Study the drawing (mm; zero at the part's minimum x, y, z) and answer. A direction names the side the tool comes from. Give positions to 0.01 mm unless a question says otherwise; leave off trailing zeros. Order: outer loops, then holes, each group sorted by start corner. A loop starts at its lowest first (then second) coordinate and runs counter-clockwise, first axis right, second up.
Item 1: Which of the six approach directions +Z, -Z, +X, -X, +Y, -Y give full straight-line access (tool end or side, diameter ignored) to the marked faces 1, 2 and 3?
Item 2: Find the intervals of material crossed by line 1 along Y through (x, z) = (3.5, 12.7); line 2 along Z through (x, y) = (3.25, 25.4); line 3 along Z through (x, y) = (17, 3), in increasing order.
Item 3: A cutting plane is placed at A-A (y = 25.4). Write down the section's boundary in (x, z), plus the area to 3 significant figures.
Item 4: A cutting plane is placed at B-B (x = 3.75). State how many separate pieces and enclosed holes the cut face has, plus the area to 3 significant figures.
Item 5: Given pin 1 Ø4 at (y, z) = (38.1, 12.7) entering from -X; pin 2 Ø6.5 at (x, z) = (12.5, 11.5) entering from -Y; pin 3 Ø7.5 at (x, z) = (16, 15) entering from +Y, each flat-ended and moving along its own axis, determine where each tip first touches the part or whether it passes through.
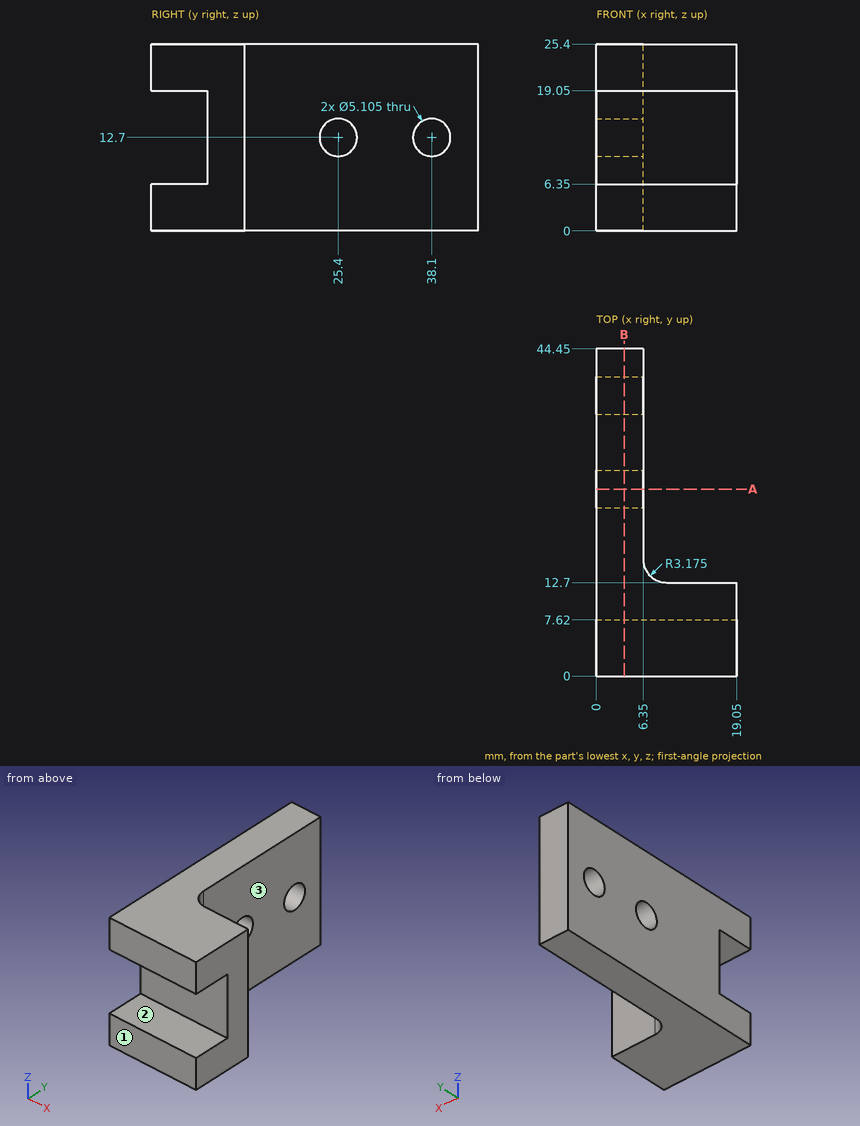
Response values:
1. face 1: +Z, -Z, +X, -X, -Y
1. face 2: +X, -X, -Y
1. face 3: +Z, -Z, +X, +Y
2. line 1: y = 7.62 to 22.85, 27.95 to 35.55, 40.65 to 44.45
2. line 2: z = 0 to 10.15, 15.25 to 25.4
2. line 3: z = 0 to 6.35, 19.05 to 25.4
3. outline: (0, 0) - (6.35, 0) - (6.35, 10.15) - (0, 10.15) - close; (0, 15.25) - (6.35, 15.25) - (6.35, 25.4) - (0, 25.4) - close
3. area: 129 mm2
4. separate pieces: 1
4. enclosed holes: 2
4. area: 991 mm2
5. pin 1: passes through
5. pin 2: stops at y = 7.62
5. pin 3: stops at y = 12.7
